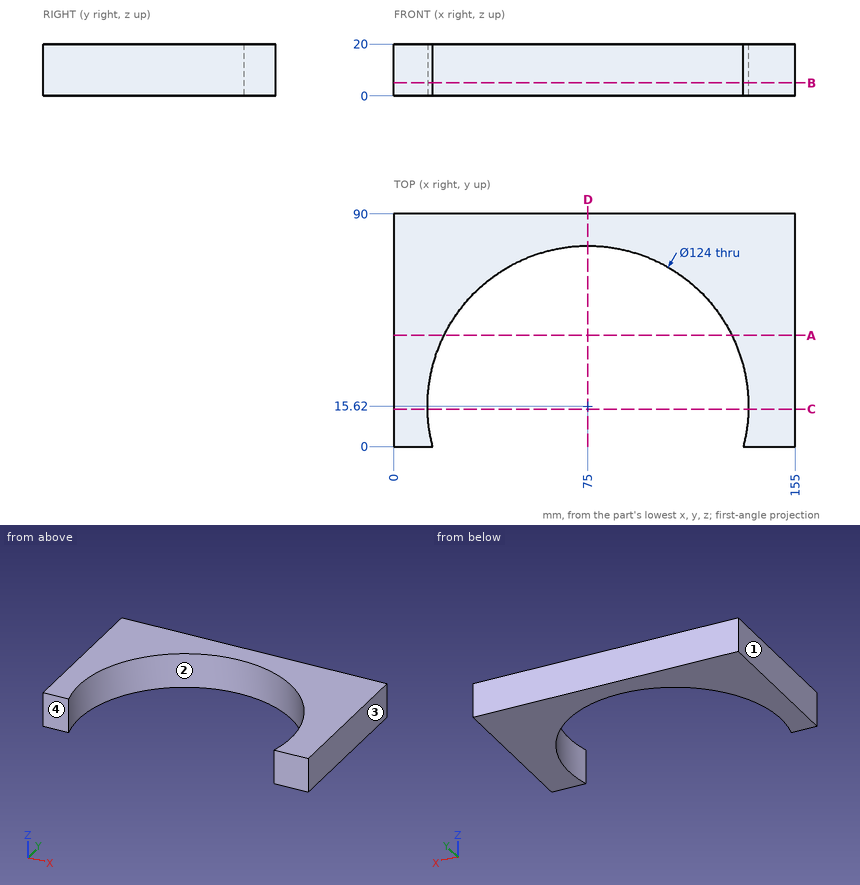
Geometry: see drawing. Coordinates: mm, zero at the bounding-box minimum. Round coordinates to 2 decimals unless told otherwise and drop trailing zeros. Order: outer loops, then holes, each group sorted by start corner. A loop starts at its lowest first (then second) coordinate and runs counter-clockwise, first axis right, second up. Notation, with made-up numbers: (80.25, -16) -> (85.25, -16) arc R22 cw to (85.25, 11) -> close; hole circle Ø11 at (84, 62.25). An arc over 180 degrees is marked (long way). Use CSV: the item, a comma, the result in double quotes.
(1) Section A-A on y = 43. Return the cut outline in (x, z).
Report:
outline,"(0, 0) -> (19.37, 0) -> (19.37, 20) -> (0, 20) -> close; (130.63, 0) -> (155, 0) -> (155, 20) -> (130.63, 20) -> close"
(2) First-contact query: pin 1 Ø1 at (x, z) = (81, 16.5) entering from -Y; pin 2 Ø8 at (x, z) = (105, 10.5) entering from -Y (1 decimal). Flat tips, straight axial feed; report the tip coordinate or a pass-through.
Report:
pin 1,"y = 77.28"
pin 2,"y = 67.5"
(3) Ray query, L1, parallel to Y at x = 77, z = 6.5; L2, parallel to X at y = 16, z = 4.25; L3, parallel to X at y = 54.5, z = 15 (1 decimal). Return the intervals inside material, ascending.
Report:
L1,"77.59 to 90"
L2,"0 to 13, 137 to 155"
L3,"0 to 26.7, 123.3 to 155"
(4) Section D-D on x = 75. Return the cut outline in (y, z), and give its area (3 significant figures).
Report:
outline,"(77.62, 0) -> (90, 0) -> (90, 20) -> (77.62, 20) -> close"
area,"248 mm^2"
(5) Pull-direction query (X, two-part tool) for the marked faces 1, 2, 3 and 4; classes: +X half, -X half, draft (parallel to the pull), parting line (faces both ways), or undercut.
Report:
face 1,"-X half"
face 2,"undercut"
face 3,"+X half"
face 4,"draft"
(6) Section C-C on y = 14.5. Return the cut outline in (x, z).
Report:
outline,"(0, 0) -> (13.01, 0) -> (13.01, 20) -> (0, 20) -> close; (136.99, 0) -> (155, 0) -> (155, 20) -> (136.99, 20) -> close"
(7) Section B-B on z = 5. Return the cut outline in (x, y).
Report:
outline,"(0, 0) -> (15, 0) arc R62 cw (long way) to (135, 0) -> (155, 0) -> (155, 90) -> (0, 90) -> close"
